Design review of the part built by this model. Coordinates are the model's own, in mm. A direction names the side the tool comes from. Coordinates: 2 decimals unless noted, no trailing zeros. Loops run counter-clockwise (first coordinate to the right, second up) from the corner with the lowest first, then second, coordinate; pieces in that order, holes last. Notation, with made-up numbers: (47, 46.25) - (75, 46.25) arc R18 ccw to (75, 68.25) - close; hole circle Ø6 at (-39.5, 57). An arc over 180 degrees is marked (long way). Answer in a Markdown table with one row per item. Add a question column.
(1) For faces 1 (the face through (19, 2, -6)), 2 (the face through (-12.5, 6, 11)), 3 (the face through (-8, 2, -6)), 4 (the face through (19, 4, 11)), 5 (the face through (7, 6, -5)), list the 3-axis set-ups (+Z, -Z, +X, -X, +Y, -Y) from which the entire face can be reached by the end or side of a thin tool; tool diameter is ignored.
(2) The part is to be moulded in two halves that separate along Z. For faces 6 (the face through (-19, 2, 0)), 7 (the face through (30, 5, 6)), 8 (the face through (3, -1, -10)), say which applies: released by +Z, released by -Z, zero draft, split by the parting line, or undercut.
(3) To check wall thickness, follow L1, parallel to X at y = 5.3, z = 11; L2, parallel to X at y = 7.75, z = 6; L3, parallel to X at y = 2, z = -8.5. State the ranges of each line that lie inside material, in increasing order. Write a range as [from, to].
(4) Clearance check with flat-ended pins moving along their axes: pin 1 (9.5 mm diameter, centred on x = 23.5, z = 13, fed in from -Y); pin 2 (3.5 mm diameter, centred on y = 2.5, z = -6, fed in from +X); pin 3 (2.5 mm diameter, centred on x = 24.5, y = 3, fed in from -Z). State where each tip first meets the part, or that it passes through.
(5) We need section C-C, the plane z = -2.5. Write out the cut boundary in (x, y).
(6) We need section A-A, the plane z = 11. Write out the cut boundary in (x, y), plus the area to 4 significant figures.
(7) We need section D-D, the plane y = 2. Write out the cut boundary in (x, z).
(8) We need section B-B, the plane x = -21.25. Write out the cut boundary in (y, z).
Autodesk Fusion 360 part; units mm, degrees
sketch "Esquisse1" plane through (0, 0, 0) normal (0, 0, 1) x (1, 0, 0)
  line L0 (30, 4) -> (-30, 4)
  line L1 (-30, 4) -> (-30, -4)
  line L2 (-30, -4) -> (30, -4)
  line L3 (30, -4) -> (30, 4)
  line L4 (30, 4) -> (-30, -4) construction
  line L5 (-30, 4) -> (30, -4) construction
  dimension "d1" = 60
  dimension "d2" = 8
extrude "Extrusion1" add sketch "Esquisse1" along normal blind 5 makes body 1
sketch "Esquisse2" plane through (0, 0, 5) normal (0, 0, 1) x (-1, 0, 0)
  line L0 (-30, 4) -> (-30, -4)
  line L1 (-30, -4) -> (30, -4)
  line L2 (30, -4) -> (30, 4)
  line L3 (30, 4) -> (-30, 4)
  line L4 (8, 4) -> (-22, 4)
  line L5 (-22, 4) -> (-22, -8)
  line L6 (-22, -8) -> (8, -8)
  line L7 (8, -8) -> (8, 4)
  line L8 (0, 12.5546) -> (0, -11.3614) construction
  line L9 (8, -2) -> (-22, -2) construction
  circle A0 centre (0, -2) radius 4
  circle A1 centre (-15, -2) radius 4
  line L10 (8, 4) -> (-22, 4)
  line L11 (0, 2) -> (-15, 2)
  line L12 (0, -6) -> (-15, -6)
  dimension "d5" = 30
  dimension "d6" = 8
  dimension "d7" = 12
  dimension "d11" = 8
  dimension "d12" = 8
  dimension "d13" = 7
extrude "Extrusion2" add sketch "Esquisse2" against normal blind 15 separate body contours L1 L3 L4 L5 L7 A0 A1 L10 L11 | L1 L5 L6 L7 A0 A1 L12 makes body 2
sketch "Esquisse3" plane through (0, 0, -10) normal (0, 0, -1) x (1, 0, 0)
  line L0 (0, 2) -> (15, 2)
  arc A0 (15, -6) -> (15, 2) centre (15, -2) ccw
  line L1 (15, -6) -> (0, -6)
  arc A1 (0, 2) -> (0, -6) centre (0, -2) ccw
  line L2 (22, 4) -> (-8, 4)
  line L3 (-8, 4) -> (-8, -8)
  line L4 (-8, -8) -> (22, -8)
  line L5 (22, -8) -> (22, 4)
  circle A2 centre (0, -2) radius 2
  circle A3 centre (15, -2) radius 4
  line L6 (0, 0) -> (11.5359, 0)
  line L7 (0, -4) -> (11.5359, -4)
  dimension "d16" = 4
  dimension "d17" = 8
extrude "Extrusion3" add sketch "Esquisse3" along normal blind 2 contours L0 L1 A1 A2 A3 L6 L7 | L2 L3 L4 L5 bodies 2
sketch "Esquisse4" plane through (0, 4, 0) normal (0, 1, 0) x (-1, 0, 0)
  line L0 (-30, 0) -> (30, 0)
  line L1 (30, 0) -> (30, 5)
  line L2 (30, 5) -> (-30, 5)
  line L3 (-30, 5) -> (-30, 0)
  line L4 (15, 10.1786) -> (15, -11.9176) construction
  line L5 (0, 1.75) -> (0, 22.5) construction
  line L6 (-30, 0) -> (-12.5, 0)
  line L7 (-12.5, 0) -> (-12.5, 17)
  line L8 (-12.5, 17) -> (-30, 17)
  line L9 (-30, 17) -> (-30, 0)
  line L10 (30, 0) -> (12.5, 0)
  line L11 (12.5, 0) -> (12.5, 17)
  line L12 (12.5, 17) -> (30, 17)
  line L13 (30, 17) -> (30, 0)
  dimension "d21" = 17
  dimension "d22" = 17
  dimension "d38" = 25
extrude "Extrusion4" add sketch "Esquisse4" along normal blind 4 contours L0 L2 L3 L6 L7 L9 | L2 L7 L8 L9 | L0 L1 L2 L10 L11 L13 | L2 L11 L12 L13 bodies 2 1
sketch "Esquisse5" plane through (0, 0, 5) normal (0, 0, 1) x (-1, 0, 0)
  arc A0 (0, -6) -> (3.4641, -4) centre (0, -2) ccw
  line L0 (0, -6) -> (-12.5, -6)
  line L1 (-12.5, -8) -> (8, -8)
  line L2 (8, -8) -> (8, -4)
  line L3 (8, -4) -> (12.5, -4)
  line L4 (12.5, -4) -> (30, -4)
  line L5 (30, -4) -> (30, 4)
  line L6 (30, 4) -> (-30, 4)
  line L7 (-30, 4) -> (-30, -4)
  line L8 (-30, -4) -> (-12.5, -4)
  line L9 (-12.5, -4) -> (3.4641, -4)
  line L10 (8, -8) -> (-22, -8)
  line L11 (-22, -8) -> (-22, -4)
  line L12 (-22, -4) -> (8, -4)
  line L13 (8, -4) -> (8, -8)
  line L14 (-12.5, -6) -> (-12.5, -8)
  point P0 (-22, 4)
extrude "Extrusion5" add sketch "Esquisse5" against normal blind 5 contours A0 L0 L8 L9 L10 L11 L12 L14 | A0 L0 L1 L2 L10 L12 L13 L14 bodies 2
sketch "Esquisse6" plane through (0, 8, 0) normal (0, 1, 0) x (-1, 0, 0)
  line L0 (30, 17) -> (12.5, 17)
  line L1 (12.5, 17) -> (12.5, 0)
  line L2 (12.5, 0) -> (30, 0)
  line L3 (30, 0) -> (30, 17)
  line L4 (30, 17) -> (12.5, 5) construction
  line L5 (12.5, 17) -> (30, 5) construction
  point P0 (21.25, 11)
  point P1 (12.5, 5)
hole "Perçage1" at (-21.25, 8, 11) direction (0, -1, 0) diameter 3 end through all countersink diameter 6 countersink angle 90 bodies 2 2
sketch "Esquisse8" plane through (0, 8, 0) normal (0, 1, 0) x (-1, 0, 0)
  line L0 (12.5, 0) -> (30, 0)
  line L1 (-30, 17) -> (-12.5, 5) construction
  line L2 (-12.5, 17) -> (-30, 5) construction
  circle A0 centre (21.25, 11) radius 3
  line L3 (30, 17) -> (12.5, 17)
  line L4 (12.5, 17) -> (12.5, 0)
  line L5 (30, 0) -> (30, 17)
  point P0 (-21.25, 11)
hole "Perçage2" at (21.25, 8, 11) direction (0, -1, 0) diameter 3 end through all countersink diameter 6 countersink angle 90 bodies 2 2
sketch "Esquisse9" plane through (-12.5, 0, 0) normal (1, 0, 0) x (0, 1, 0)
  line L0 (4, 5) -> (4, 0)
  line L1 (4, 0) -> (8, 0)
  line L2 (8, 0) -> (8, 17)
  line L3 (8, 17) -> (4, 17)
  line L4 (4, 17) -> (4, 5)
  line L5 (8, 0) -> (4, 0)
  line L6 (4, 0) -> (4, 5)
  line L7 (4, 5) -> (8, 5)
  line L8 (8, 5) -> (8, 0)
extrude "Extrusion6" add sketch "Esquisse9" along normal up to surface (4.5 mm away) contours L0 L1 L2 L5 L6 L7 L8 bodies 2
Responses:
| question | item | result |
|---|---|---|
| 1 | face 1 | -Z |
| 1 | face 2 | +Z, +Y, -Y |
| 1 | face 3 | -Z, -X, +Y, -Y |
| 1 | face 4 | +Z, +X, -X, -Y |
| 1 | face 5 | none |
| 2 | face 6 | released by -Z |
| 2 | face 7 | zero draft |
| 2 | face 8 | undercut |
| 3 | L1 | x = [-30, -22.75], [-19.75, -12.5], [12.5, 19.75], [22.75, 30] |
| 3 | L2 | x = [-30, -12.5], [12.5, 30] |
| 3 | L3 | x = [-8, -4], [19, 22] |
| 4 | pin 1 | stops at y = 4 |
| 4 | pin 2 | stops at x = 22 |
| 4 | pin 3 | stops at z = 0 |
| 5 | outline | (-8, -4) - (22, -4) - (22, 8) - (-8, 8) - close; hole (0, -2) - (15, -2) arc R4 ccw to (15, 6) - (0, 6) arc R4 ccw to start |
| 6 | outline | (-30, 4) - (-22.75, 4) - (-22.75, 6.5) - (-24.25, 8) - (-30, 8) - close; (-19.75, 4) - (-12.5, 4) - (-12.5, 8) - (-18.25, 8) - (-19.75, 6.5) - close; (12.5, 4) - (19.75, 4) - (19.75, 6.5) - (18.25, 8) - (12.5, 8) - close; (22.75, 4) - (30, 4) - (30, 8) - (24.25, 8) - (22.75, 6.5) - close |
| 6 | area | 111.5 mm2 |
| 7 | outline | (-30, 0) - (-8, 0) - (-8, -12) - (-2, -12) - (-2, -10) - (-4, -10) - (-4, 0) - (19, 0) - (19, -12) - (22, -12) - (22, 0) - (30, 0) - (30, 5) - (-30, 5) - close |
| 8 | outline | (-4, 0) - (8, 0) - (8, 8) - (6.5, 9.5) - (4, 9.5) - (4, 5) - (-4, 5) - close; (4, 12.5) - (6.5, 12.5) - (8, 14) - (8, 17) - (4, 17) - close |
